```python
from build123d import *

# Parameters (mm, degrees)
F0_W     = 100
F0_H     = 63
F1_DEPTH = 12
F2_R     = 3
F3_DEPTH = 11.5
F4_R     = 3
F5_DEPTH = 12.001


with BuildPart() as f1:
    # F0 (on Front) → F1 (new body)
    with BuildSketch(Plane.XZ):
        with Locations((50, 31.5)):
            Rectangle(F0_W, F0_H)
    extrude(amount=F1_DEPTH)

    # F2 (on face) → F3 (join)
    with BuildSketch(Plane(origin=(0, 0, 0), x_dir=(1, 0, 0), z_dir=(0, 0, -1))):
        with Locations((7.5, 6)):
            Circle(F2_R)
        with Locations((92.5, 6)):
            Circle(F2_R)
    extrude(amount=F3_DEPTH)

    # F4 (on face) → F5 (cut, through all)
    with BuildSketch(Plane.XZ.offset(12)):
        with Locations((75, 38)):
            Circle(F4_R)
    extrude(amount=-F5_DEPTH, mode=Mode.SUBTRACT)


solid = f1.part
```
Verification items for the finished model (mm, model axes). A direction names the side the tool comes from. Coordinates: 2 decimals unless noted, no trailing zeros. Loops run counter-clockwise (first coordinate to the right, second up) from the corner with the lowest first, then second, coordinate; pieces in that order, holes last. Notation, with made-up numbers: (54.5, 38) - (71.5, 38) arc R23 cw to (71.5, 61) - close; hole circle Ø8 at (44.25, 27). An arc over 180 degrees is marked (long way). Answer as a JSON object with one key per item and string values.
(1) Cross-section at C-C, the plane z = 38. Record the boundary of the cut face in (x, y), then the cut area to 3 significant figures.
Response:
{"outline": "(0, -12) - (72, -12) - (72, 0) - (0, 0) - close; (78, -12) - (100, -12) - (100, 0) - (78, 0) - close", "area": "1,130 mm²"}
(2) Scan lines: line 1 along Z through (x, y) = (75, -8); line 2 along Z through (x, y) = (16, -0.5); line 3 along X through (y, z) = (-6, -7.5). Record each from-to range of solid material in increasing order.
Response:
{"line 1": "z = 0 to 35, 41 to 63", "line 2": "z = 0 to 63", "line 3": "x = 4.5 to 10.5, 89.5 to 95.5"}
(3) Cross-section at A-A, the plane x = 75. Record the boundary of the cut face in (y, z), then the cut area to 3 significant figures.
Response:
{"outline": "(-12, 0) - (0, 0) - (0, 35) - (-12, 35) - close; (-12, 41) - (0, 41) - (0, 63) - (-12, 63) - close", "area": "684 mm²"}
(4) Cross-section at B-B, the plane y = -6. Record the boundary of the cut face in (x, z).
Response:
{"outline": "(0, 0) - (4.5, 0) - (4.5, -11.5) - (10.5, -11.5) - (10.5, 0) - (89.5, 0) - (89.5, -11.5) - (95.5, -11.5) - (95.5, 0) - (100, 0) - (100, 63) - (0, 63) - close; hole circle Ø6 at (75, 38)"}
(5) Go/stop test with flat-tipped pins: pin 1 Ø5 at (x, z) = (75, 38) entering from +Y; pin 2 Ø6 at (x, y) = (68.5, -2) entering from -Z. Record where each tip stops, or that it passes through.
Response:
{"pin 1": "passes through", "pin 2": "stops at z = 0"}
(6) Access from +Z, -Z, +X, -X, +Y, -Y to the whole of each face (thin tool, end or side, straight path). Record for faces 1 (the cylindrical face through (89.5, -6.1, -5.7)), 2 (the flat face through (49, 0, 32)).
Response:
{"face 1": "-Z", "face 2": "+Z, -Z, +X, -X, +Y"}
(7) Cross-section at D-D, the plane x = 7.5. Record the boundary of the cut face in (y, z), then the cut area to 3 significant figures.
Response:
{"outline": "(-12, 0) - (-9, 0) - (-9, -11.5) - (-3, -11.5) - (-3, 0) - (0, 0) - (0, 63) - (-12, 63) - close", "area": "825 mm²"}
(8) Mould release check, pull along X, two halves, no side actions. Record for faces 3 (the cylindrical face through (10.27, -4.85, -5.67)), 4 (the flat face through (100, -6, 31)), 5 (the flat face through (49, -6, 63)): pulls with the +X half, pulls with the -X half, needs draft (parallel to the pull), parting line crosses it, or undercut.
Response:
{"face 3": "undercut", "face 4": "pulls with the +X half", "face 5": "needs draft"}
